Build history of the part. All positions in model axes, mm. A direction names the side the tool comes from. Give positions to 0.01 mm unless a question says otherwise; leave off trailing zeros. Write each loop counter-clockwise with the first axis right and the second up, starting at its lowest first coordinate (ties: lowest second). Pieces come first, ordered by that corner, then holes. Notation, with made-up numbers: M 39.5,68 L 51.5,68 A16 cw 51.5,80 Z; hole C -3,-14.5 d1. An arc over 180 degrees is marked long. Return JSON: item names as keys, results as strings. Group by question number.
Q1. Flat gauge pins, fed straight in: pin 1 Ø1.5 at (y, z) = (1, -7.5) entering from +X; pin 2 Ø0.9 at (y, z) = (0.5, 1) entering from +X; pin 3 Ø1.5 at (y, z) = (-1.5, -0.5) entering from +X. Where does each tip first touch, or does it go through?
Q2. Band-saw the part on A-A, the plane z = -1. Give the cut face in (x, y).
Q3. Wall check: probe 1 along Z at (x, y) = (-0.2, -0.05); probe 2 along X at (y, z) = (-0.65, 1); probe 3 along Z at (x, y) = (1.2, -2.1). Give the ranges that are in metal, low to high.
Q4. Pull direction X, two halves, no side cores. Call faces 3 (the cylindrical face through (1.5, 0.07, -4.78)), 4 (the flat face through (0, 0, -10)), 5 (the flat face through (0, 0, -0.35)): +X half, -X half, draft (parallel to the pull), parting line (faces both ways), or undercut.
Q5. Tool access for faces 1 (the flat face through (-1, 0, 1)), 2 (the flat face through (1.2, -1.2, 0)): list every direction of +Z, -Z, +X, -X, +Y, -Y with a clear straight run to the whole face (end or side of a thin tool).
from build123d import *

# Parameters (mm, degrees)
SKETCH1_R           = 2.85
BOSS_EXTRUDE1_DEPTH = 1.65
SKETCH2_R           = 1.5
BOSS_EXTRUDE2_DEPTH = 10
CHAMFER1_SIZE       = 0.3
CUT_EXTRUDE1_DEPTH  = 2
FILLET1_R           = 1.5


with BuildPart() as part:
    # Sketch1 → Boss-Extrude1 (new body)
    with BuildSketch(Plane.XY):
        Circle(SKETCH1_R)
    extrude(amount=BOSS_EXTRUDE1_DEPTH)

    # Sketch2 → Boss-Extrude2 (add)
    with BuildSketch(Plane(origin=(0, 0, 0), x_dir=(-1, 0, 0), z_dir=(0, 0, -1))):
        Circle(SKETCH2_R)
    extrude(amount=BOSS_EXTRUDE2_DEPTH)

    # Chamfer1
    chamfer1_edges = [part.edges().sort_by_distance(p)[0] for p in [
        (1.5, 0, -10),
    ]]
    chamfer(chamfer1_edges, length=CHAMFER1_SIZE)

    # Sketch3 → Cut-Extrude1 (cut)
    with BuildSketch(Plane.XY.offset(1.65)):
        Polygon((0, 1.154700538), (-1, 0.577350269), (-1, -0.577350269), (0, -1.154700538), (1, -0.577350269), (1, 0.577350269), align=None)
    extrude(amount=-CUT_EXTRUDE1_DEPTH, mode=Mode.SUBTRACT)

    # Fillet1
    fillet1_edges = [part.edges().sort_by_distance(p)[0] for p in [
        (-2.85, 0, 1.65),
    ]]
    fillet(fillet1_edges, radius=FILLET1_R)


solid = part.part
From the geometry:
{
 "1": {"pin 1": "stops at x = 1.48", "pin 2": "stops at x = 2.77", "pin 3": "stops at x = 2.69"},
 "2": {"outline": "C 0,0 d3"},
 "3": {"probe 1": "z = -10 to -0.35", "probe 2": "x = -2.5 to -0.87, 0.87 to 2.5", "probe 3": "z = 0 to 1.2"},
 "4": {"face 3": "parting line", "face 4": "draft", "face 5": "undercut"},
 "5": {"face 1": "+Z", "face 2": "-Z"}
}
